```python
from build123d import *

# Parameters (mm, degrees)
SKETCH_R      = 30.15
PAD_DEPTH     = 60
SKETCH001_R   = 24.15
POCKET_DEPTH  = 48
SKETCH002_R   = 24
SKETCH002_R_2 = 9.5
PAD001_DEPTH  = 10
SKETCH003_R   = 24
SKETCH003_R_2 = 9.5
PAD002_DEPTH  = 10


with BuildPart() as part:
    # Sketch → Pad (new body)
    with BuildSketch(Plane.XY):
        Circle(SKETCH_R)
    extrude(amount=PAD_DEPTH)

    # Sketch001 (on Face2 of Pad) → Pocket (cut)
    with BuildSketch(Plane(origin=(0, 0, 0), x_dir=(1, 0, 0), z_dir=(0, 0, -1))):
        Circle(SKETCH001_R)
    extrude(amount=-POCKET_DEPTH, mode=Mode.SUBTRACT)

    # Sketch002 → Pad001 (join)
    with BuildSketch(Plane.XZ.offset(5)):
        with Locations((0, 80)):
            Circle(SKETCH002_R)
        with Locations((0, 80)):
            Circle(SKETCH002_R_2, mode=Mode.SUBTRACT)
    extrude(amount=PAD001_DEPTH)

    # Sketch003 → Pad002 (join)
    with BuildSketch(Plane.XZ.offset(-5)):
        with Locations((0, 80)):
            Circle(SKETCH003_R)
        with Locations((0, 80)):
            Circle(SKETCH003_R_2, mode=Mode.SUBTRACT)
    extrude(amount=-PAD002_DEPTH)


solid = part.part
```
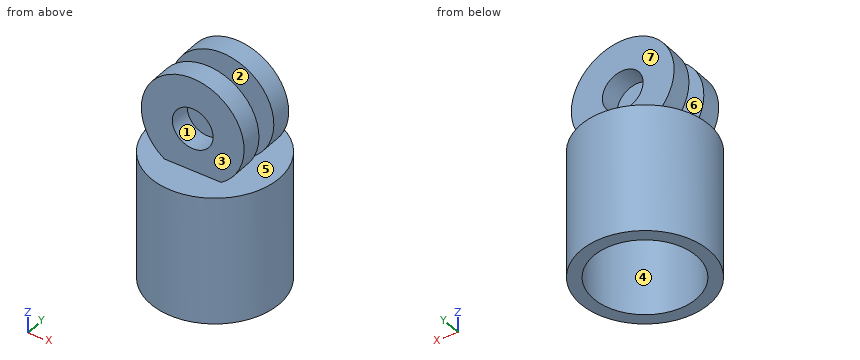
Source: CAD feature listing. Evaluate the final solid. Frame: model axes, mm. Face numbers are marked on the shaded views. A direction names the side the tool comes from. Give positions to 0.01 mm unless a question says otherwise; leave off trailing zeros. Loops run counter-clockwise (first coordinate to the right, second up) from the corner with the lowest first, then second, coordinate; pieces in that order, holes last. Notation, with made-up numbers: (55, 35.25) - (60, 35.25) arc R13 cw to (60, 51.25) - close; hole circle Ø9 at (4, 33.5). An arc over 180 degrees is marked (long way). Use CSV: the item, a comma, the result in double quotes.
1) Mould query, pull axis Y, two halves, no side actions, for the marked faces 1, 2, 3 and 4. Classes: +Y half, -Y half, draft (parallel to the pull), parting line (faces both ways), or undercut.
Worked out:
face 1,"draft"
face 2,"undercut"
face 3,"-Y half"
face 4,"undercut"
2) Cut plane A-A (x = 0). Output: boundary loops of the cut face in (y, z), and give its area (3 significant figures).
Worked out:
outline,"(-30.15, 0) - (-24.15, 0) - (-24.15, 48) - (24.15, 48) - (24.15, 0) - (30.15, 0) - (30.15, 60) - (15, 60) - (15, 70.5) - (5, 70.5) - (5, 60) - (-5, 60) - (-5, 70.5) - (-15, 70.5) - (-15, 60) - (-30.15, 60) - close; (-15, 89.5) - (-5, 89.5) - (-5, 104) - (-15, 104) - close; (5, 89.5) - (15, 89.5) - (15, 104) - (5, 104) - close"
area,"1,800 mm^2"
3) Cut plane C-C (y = 0). Output: boundary loops of the cut face in (x, z).
Worked out:
outline,"(-30.15, 0) - (-24.15, 0) - (-24.15, 48) - (24.15, 48) - (24.15, 0) - (30.15, 0) - (30.15, 60) - (-30.15, 60) - close"
4) Pin query (flat end, axial travel): P1, Ø22, axis at x = 0, z = 80, coming from the -Y side; P2, Ø2, axis at x = 9.5, y = -3.5, coming from the +Z side; P3, Ø22, axis at x = 3.5, z = 92, coming from the +Y side; P4, Ø8, axis at y = -1.5, z = 47, coming from the +X side. Return the tip coordinate at first contact, or that it passes through.
Worked out:
P1,"stops at y = -15"
P2,"stops at z = 60"
P3,"stops at y = 15"
P4,"stops at x = 30.15"
5) Cut plane D-D (z = 23.5). Output: boundary loops of the cut face in (x, y).
Worked out:
outline,"circle Ø60.3 at (0, 0); hole circle Ø48.3 at (0, 0)"
6) Set-up query: the marked faces 5, 6 and 7. Return all of +Z, -Z, +X, -X, +Y, -Y with unobstructed straight access to the full face (end or side cutting, diameter ignored); none if empty.
Worked out:
face 5,"none"
face 6,"+Z, +X, -X"
face 7,"+Z, +X, -X, +Y"
7) Line query: line 1 (Y direction, x = 0, z = 10); line 2 (Z direction, x = 0, y = 9); line 3 (Z direction, x = -8.5, y = 22). Output: solid intervals per line, ascending.
Worked out:
line 1,"y = -30.15 to -24.15, 24.15 to 30.15"
line 2,"z = 48 to 70.5, 89.5 to 104"
line 3,"z = 48 to 60"
8) Cut plane B-B (z = 80). Output: boundary loops of the cut face in (x, y).
Worked out:
outline,"(-24, -15) - (-9.5, -15) - (-9.5, -5) - (-24, -5) - close; (-24, 5) - (-9.5, 5) - (-9.5, 15) - (-24, 15) - close; (9.5, -15) - (24, -15) - (24, -5) - (9.5, -5) - close; (9.5, 5) - (24, 5) - (24, 15) - (9.5, 15) - close"
